Design review of the part built by this model. Coordinates are the model's own, in mm. Face numbers are marked on the shaded views. A direction names the side the tool comes from. Give positions to 0.01 mm unless a question says otherwise; leave off trailing zeros. Loops run counter-clockwise (first coordinate to the right, second up) from the corner with the lowest first, then second, coordinate; pieces in that order, holes last.
from build123d import *

# Parameters (mm, degrees)
F0_W     = 50
F0_H     = 40
F1_DEPTH = 30
F2_W     = 25
F2_H     = 30
F3_DEPTH = 50.001
F4_W     = 25
F4_H     = 25
F5_DEPTH = 30.001
F7_DEPTH = 40.001


with BuildPart() as f1:
    # F0 (on Top) → F1 (new body)
    with BuildSketch(Plane.XY):
        Rectangle(F0_W, F0_H)
    extrude(amount=F1_DEPTH)

    # F2 (on face) → F3 (cut, through all)
    with BuildSketch(Plane.YZ.offset(25)):
        Rectangle(F2_W, F2_H)
    extrude(amount=-F3_DEPTH, mode=Mode.SUBTRACT)

    # F4 (on face) → F5 (cut, through all)
    with BuildSketch(Plane.XY.offset(30)):
        Rectangle(F4_W, F4_H)
    extrude(amount=-F5_DEPTH, mode=Mode.SUBTRACT)

    # F6 (on face) → F7 (cut, through all)
    with BuildSketch(Plane(origin=(0, 20, 0), x_dir=(-1, 0, 0), z_dir=(0, 1, 0))):
        Polygon((2, 30), (0, 30), (-2, 30), (0, 28), align=None)
    extrude(amount=-F7_DEPTH, mode=Mode.SUBTRACT)


solid = f1.part
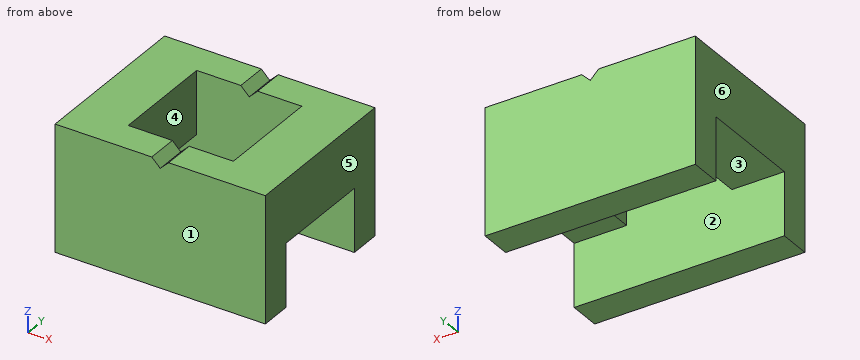
Q1. Take a section at D-D (x = 18.5). Give the boundary of the cut face in (y, z).
Results:
outline: (-20, 0) - (-12.5, 0) - (-12.5, 15) - (12.5, 15) - (12.5, 0) - (20, 0) - (20, 30) - (-20, 30) - close
Q2. Insertion check: pin 1 (4 mm diameter, centred on x = 20.5, y = -5, fed in from -Z); pin 2 (5 mm diameter, centred on y = -9.5, z = 11.5, fed in from +X). Each pin has a flat end and moves straight along its axis. Give the tip position at first contact, or say it passes through.
Results:
pin 1: stops at z = 15
pin 2: passes through
Q3. Take a section at A-A (x = 7.5). Give the boundary of the cut face in (y, z).
Results:
outline: (-20, 0) - (-12.5, 0) - (-12.5, 30) - (-20, 30) - close; (12.5, 0) - (20, 0) - (20, 30) - (12.5, 30) - close
Q4. Draft analysis for pull direction X (two halves, no side actions). For the marked faces 4, 5 and 6, state which applies: pulls with the +X half, pulls with the -X half, needs draft (parallel to the pull), parting line crosses it, or undercut.
Results:
face 4: undercut
face 5: pulls with the +X half
face 6: pulls with the -X half
Q5. Tool access review of the marked faces 1, 2 and 3: name each direction out of +Z, -Z, +X, -X, +Y, -Y from which nothing blocks a thin tool from reaching the whole face with its end or side.
Results:
face 1: +Z, -Z, +X, -X, -Y
face 2: -Z
face 3: -Z, +X, -X
Q6. Take a section at B-B (y = -7). Give the boundary of the cut face in (x, z), plus the area to 3 significant figures.
Results:
outline: (-25, 15) - (-12.5, 15) - (-12.5, 30) - (-25, 30) - close; (12.5, 15) - (25, 15) - (25, 30) - (12.5, 30) - close
area: 375 mm2
Q7. Take a section at C-C (z = 25.5). Give the boundary of the cut face in (x, y).
Results:
outline: (-25, -20) - (25, -20) - (25, 20) - (-25, 20) - close; hole (-12.5, -12.5) - (12.5, -12.5) - (12.5, 12.5) - (-12.5, 12.5) - close
Q8. Wall thickness on line 1 (Y direction, x = 7.5, z = 26.5); line 2 (X direction, y = 8.5, z = 18); line 3 (Z direction, x = -13.5, y = -11.5): over which ranges is each line inside the solid? List them lowest first.
Results:
line 1: y = -20 to -12.5, 12.5 to 20
line 2: x = -25 to -12.5, 12.5 to 25
line 3: z = 15 to 30
